Verification items for the finished model (mm, model axes). A direction names the side the tool comes from. Round coordinates to 2 decimals unless told otherwise and drop trailing zeros. Loops run counter-clockwise (first coordinate to the right, second up) from the corner with the lowest first, then second, coordinate; pieces in that order, holes last. Notation, with made-up numbers: (44, 83) -> (70, 83) arc R19 cw to (70, 88) -> close; hole circle Ø8 at (-2.5, 69). An arc over 180 degrees is marked (long way). Use a Markdown table: item, result. Add a question column.
```python
from build123d import *

# Parameters (mm, degrees)
SKETCH_1_R      = 4.1
EXTRUDE_1_DEPTH = 10


with BuildPart() as part:
    # 草圖1 → 填料-伸長1 (new body)
    with BuildSketch(Plane.XY):
        with BuildLine():
            Line((-50, 0), (-35, 0))
            Line((-35, 0), (-35, -5))
            Line((-35, -5), (-15, -5))
            Line((-15, -5), (-15, 0))
            Line((-15, 0), (15, 0))
            Line((15, 0), (15, -5))
            Line((15, -5), (35, -5))
            Line((35, -5), (35, 0))
            Line((35, 0), (50, 0))
            Line((50, 0), (50, 299))
            ThreePointArc((50, 299), (0, 349), (-50, 299))
            Line((-50, 299), (-50, 0))
        make_face()
        with Locations((0, 299)):
            Circle(SKETCH_1_R, mode=Mode.SUBTRACT)
        with Locations((0, 28.5)):
            Circle(SKETCH_1_R, mode=Mode.SUBTRACT)
    extrude(amount=-EXTRUDE_1_DEPTH)


solid = part.part
```
1) Access from +Z, -Z, +X, -X, +Y, -Y to the whole of each face (thin tool, end or side, straight path). Record for faces 4 (the face through (0, 0, -5)), 5 (the face through (42, 0, -5)), 6 (the face through (-50, 152, -5)).
2) Sectioned sample at C-C on z = -8.5. Enter the section's corners in (x, y), then the cut area to 3 significant figures.
3) Sectioned sample at B-B on x = 0. Enter the section's corners in (y, z), then the cut area to 3 significant figures.
4) Sectioned sample at D-D on x = 39.5. Enter the section's corners in (y, z).
5) Thickness scan on line 1 (Y direction, x = 0, z = -3.5); line 2 (X direction, y = 299, z = -3.5); line 3 (Y direction, x = -46, z = -1.25). Record the ranges inside material, lowest first.
6) Go/stop test with flat-tipped pins: pin 1 (5 mm diameter, centred on x = -41, z = -7, fed in from -Y); pin 2 (3 mm diameter, centred on x = 13.5, z = -5.5, fed in from +Y); pin 3 (1.5 mm diameter, centred on y = -2, z = -7, fed in from +X). Record where each tip stops, or that it passes through.
7) Release check for a two-part mould opening along Y. For faces 1 (the face through (-43, 0, -5)), 2 (the face through (50, 147, -5)), 3 (the face through (-0.534, 303.065, -4.93)) record: released by +Y, released by -Y, zero draft, split by the parting line, or undercut.
8) Sectioned sample at A-A on y = 28.5. Enter the section's corners in (x, z).
Geometry results:
| question | item | result |
|---|---|---|
| 1 | face 4 | +Z, -Z, -Y |
| 1 | face 5 | +Z, -Z, +X, -Y |
| 1 | face 6 | +Z, -Z, -X, +Y, -Y |
| 2 | outline | (-50, 0) -> (-35, 0) -> (-35, -5) -> (-15, -5) -> (-15, 0) -> (15, 0) -> (15, -5) -> (35, -5) -> (35, 0) -> (50, 0) -> (50, 299) arc R50 ccw to (-50, 299) -> close; hole circle Ø8.2 at (0, 28.5); hole circle Ø8.2 at (0, 299) |
| 2 | area | 33,900 mm^2 |
| 3 | outline | (0, -10) -> (24.4, -10) -> (24.4, 0) -> (0, 0) -> close; (32.6, -10) -> (294.9, -10) -> (294.9, 0) -> (32.6, 0) -> close; (303.1, -10) -> (349, -10) -> (349, 0) -> (303.1, 0) -> close |
| 3 | area | 3,330 mm^2 |
| 4 | outline | (0, -10) -> (329.66, -10) -> (329.66, 0) -> (0, 0) -> close |
| 5 | line 1 | 0 to 24.4, 32.6 to 294.9, 303.1 to 349 |
| 5 | line 2 | -50 to -4.1, 4.1 to 50 |
| 5 | line 3 | 0 to 318.6 |
| 6 | pin 1 | y = 0 |
| 6 | pin 2 | y = 347.54 |
| 6 | pin 3 | x = 35 |
| 7 | face 1 | released by -Y |
| 7 | face 2 | zero draft |
| 7 | face 3 | undercut |
| 8 | outline | (-50, -10) -> (-4.1, -10) -> (-4.1, 0) -> (-50, 0) -> close; (4.1, -10) -> (50, -10) -> (50, 0) -> (4.1, 0) -> close |
